Autodesk Inventor part; units mm, degrees
ref_plane "YZ Plane" through (0, 0, 0) normal (1, 0, 0) x (0, 1, 0)
ref_plane "XZ Plane" through (0, 0, 0) normal (0, 1, 0) x (-1, 0, 0)
ref_plane "XY Plane" through (0, 0, 0) normal (0, 0, 1) x (1, 0, 0)
sketch "Sketch1" plane through (0, 0, 0) normal (1, 0, 0) x (0, 1, 0)
  arc A0 (19.1422, -3.9768) -> (18.6646, -2.8408) centre (18.6646, -3.5092) ccw
  line L0 (15.9535, -7.2342) -> (19.1422, -3.9768)
  line L1 (21.0667, -5.7702) -> (17.9387, -8.9655)
  arc A1 (22.2128, -6.2377) -> (21.0667, -5.7702) centre (21.5444, -6.2377) ccw
  line L2 (25.0536, -2.0053) -> (25.0536, -8.7443)
  line L3 (22.2128, -8.7443) -> (22.2128, -6.2377)
  line L4 (-0.0122, -2.0053) -> (-0.0122, -8.7443)
  arc A2 (3.9747, -5.7702) -> (2.8286, -6.2377) centre (3.497, -6.2377) ccw
  arc A3 (1.9931, 0) -> (-0.0122, -2.0053) centre (1.9931, -2.0053) ccw
  line L5 (8.8992, 0) -> (1.9931, 0)
  arc A4 (7.1027, -16.4345) -> (8.0089, -14.2135) centre (4.8339, -14.2135) ccw
  arc A5 (18.6646, -22.5592) -> (19.1422, -21.4232) centre (18.6646, -21.8908) ccw
  line L6 (15.9535, -18.1658) -> (19.1422, -21.4232)
  arc A6 (21.0667, -19.6298) -> (22.2128, -19.1623) centre (21.5444, -19.1623) ccw
  line L7 (21.0667, -19.6298) -> (17.9387, -16.4345)
  line L8 (22.2128, -16.6557) -> (22.2128, -19.1623)
  line L9 (25.0536, -23.3947) -> (25.0536, -16.6557)
  line L10 (16.1422, 0) -> (23.0483, 0)
  line L11 (18.6646, -2.8408) -> (16.0299, -2.8408)
  arc A7 (22.2128, -8.7443) -> (23.3277, -9.8592) centre (23.3277, -8.7443) ccw
  line L12 (23.9387, -9.8592) -> (23.3277, -9.8592)
  arc A8 (23.9387, -9.8592) -> (25.0536, -8.7443) centre (23.9387, -8.7443) ccw
  arc A9 (6.3768, -2.8408) -> (5.8991, -3.9768) centre (6.3768, -3.5092) ccw
  line L13 (3.9747, -5.7702) -> (7.1027, -8.9655)
  line L14 (9.0879, -7.2342) -> (5.8991, -3.9768)
  arc A10 (2.8286, -19.1623) -> (3.9747, -19.6298) centre (3.497, -19.1623) ccw
  line L15 (-0.0122, -23.3947) -> (-0.0122, -16.6557)
  line L16 (3.9747, -19.6298) -> (7.1027, -16.4345)
  arc A11 (5.8991, -21.4232) -> (6.3768, -22.5592) centre (6.3768, -21.8908) ccw
  line L17 (9.0879, -18.1658) -> (5.8991, -21.4232)
  line L18 (2.8286, -16.6557) -> (2.8286, -19.1623)
  arc A12 (23.0483, -25.4) -> (25.0536, -23.3947) centre (23.0483, -23.3947) ccw
  arc A13 (25.0536, -2.0053) -> (23.0483, 0) centre (23.0483, -2.0053) ccw
  arc A14 (13.6846, -8.1882) -> (15.9535, -7.2342) centre (13.6846, -5.0132) ccw
  line L19 (13.6846, -8.1882) -> (11.3567, -8.1882)
  arc A15 (9.0115, -2.8408) -> (10.0141, -1.8382) centre (9.0115, -1.8382) ccw
  arc A16 (9.0879, -7.2342) -> (11.3567, -8.1882) centre (11.3567, -5.0132) ccw
  arc A17 (17.9387, -8.9655) -> (17.0325, -11.1865) centre (20.2075, -11.1865) ccw
  line L20 (17.0325, -14.2135) -> (17.0325, -11.1865)
  line L21 (6.3768, -2.8408) -> (9.0115, -2.8408)
  line L22 (10.0141, -1.8382) -> (10.0141, -1.1149)
  arc A18 (10.0141, -1.1149) -> (8.8992, 0) centre (8.8992, -1.1149) ccw
  line L23 (2.8286, -8.7443) -> (2.8286, -6.2377)
  arc A19 (1.7137, -9.8592) -> (2.8286, -8.7443) centre (1.7137, -8.7443) ccw
  line L24 (1.1027, -9.8592) -> (1.7137, -9.8592)
  arc A20 (-0.0122, -8.7443) -> (1.1027, -9.8592) centre (1.1027, -8.7443) ccw
  line L25 (6.3768, -22.5592) -> (9.0115, -22.5592)
  arc A21 (10.0141, -23.5618) -> (9.0115, -22.5592) centre (9.0115, -23.5618) ccw
  line L26 (10.0141, -23.5618) -> (10.0141, -24.2851)
  arc A22 (8.8992, -25.4) -> (10.0141, -24.2851) centre (8.8992, -24.2851) ccw
  line L27 (8.8992, -25.4) -> (1.9931, -25.4)
  arc A23 (17.0325, -14.2135) -> (17.9387, -16.4345) centre (20.2075, -14.2135) ccw
  line L28 (23.9387, -15.5408) -> (23.3277, -15.5408)
  arc A24 (23.3277, -15.5408) -> (22.2128, -16.6557) centre (23.3277, -16.6557) ccw
  arc A25 (25.0536, -16.6557) -> (23.9387, -15.5408) centre (23.9387, -16.6557) ccw
  line L29 (16.1422, -25.4) -> (23.0483, -25.4)
  line L30 (18.6646, -22.5592) -> (16.0299, -22.5592)
  line L31 (8.0089, -11.1865) -> (8.0089, -14.2135)
  arc A26 (8.0089, -11.1865) -> (7.1027, -8.9655) centre (4.8339, -11.1865) ccw
  arc A27 (15.0273, -1.8382) -> (16.0299, -2.8408) centre (16.0299, -1.8382) ccw
  line L32 (15.0273, -1.8382) -> (15.0273, -1.1149)
  arc A28 (16.1422, 0) -> (15.0273, -1.1149) centre (16.1422, -1.1149) ccw
  arc A29 (-0.0122, -23.3947) -> (1.9931, -25.4) centre (1.9931, -23.3947) ccw
  arc A30 (11.3567, -17.2118) -> (9.0879, -18.1658) centre (11.3567, -20.3868) ccw
  line L33 (11.3567, -17.2118) -> (13.6846, -17.2118)
  arc A31 (15.9535, -18.1658) -> (13.6846, -17.2118) centre (13.6846, -20.3868) ccw
  arc A32 (16.0299, -22.5592) -> (15.0273, -23.5618) centre (16.0299, -23.5618) ccw
  line L34 (15.0273, -23.5618) -> (15.0273, -24.2851)
  arc A33 (15.0273, -24.2851) -> (16.1422, -25.4) centre (16.1422, -24.2851) ccw
  line L35 (1.1027, -15.5408) -> (1.7137, -15.5408)
  arc A34 (1.1027, -15.5408) -> (-0.0122, -16.6557) centre (1.1027, -16.6557) ccw
  arc A35 (2.8286, -16.6557) -> (1.7137, -15.5408) centre (1.7137, -16.6557) ccw
  point P0 (0, 0)
  point P1 (12.5207, -12.7)
  dimension "d0" = 25.4
extrude "Extrusion1" add sketch "Sketch1" along normal blind 101.6
properties part number "extruded aluminum"
Model file for the job. Use its own axes, mm. A direction names the side the tool comes from. Coordinates: 2 decimals unless noted, no trailing zeros. Write each loop counter-clockwise with the first axis right and the second up, starting at its lowest first coordinate (ties: lowest second). Pieces come first, ordered by that corner, then holes. Notation, with made-up numbers: (69, -22.5) - (119, -22.5) arc R10 cw to (119, -10.5) - close; hole circle Ø11 at (-28.75, 16). An arc over 180 degrees is marked (long way). One line per question, with ' | ' between items. Start each with the question number.
Q1. Pull direction Z, two halves, no side cores. Call faces 4 (the face through (50, 20, -25.4)), 5 (the face through (50, -0.012, -20)), 6 (the face through (50.09, 19.52, -7.35)): pulls with the +Z half, pulls with the -Z half, needs draft (parallel to the pull), parting line crosses it, or undercut.
Q2. Cut at A-A, the plane z = -12.25. List the corners of the cut face in (x, y), then the cut area to 3 significant figures.
Q3. Drill centre lines: line 1 (Z direction, x = 5.5, y = 3.5); line 2 (Z direction, x = 43, y = 7.5); line 3 (Z direction, x = 73.5, y = 16.25). Where is each one in solid material? Low to high. Write a range as [from, to].
Q4. 3-axis set-ups, long thin cutter, end or side, ignore diameter. For faces 1 (the face through (50, 17.032, -13)), 2 (the face through (50, 13, -17.212)), 3 (the face through (50.089, 17.274, -15.429)): which of +Z, -Z, +X, -X, +Y, -Y reach the whole face in a straight line?
Q5. Pin check, flat tips, straight feed: pin 1 (0.6 mm diameter, centred on x = 58.5, z = -1.5, fed in from -Y); pin 2 (2.5 mm diameter, centred on x = 69, z = -13, fed in from -Y); pin 3 (0.5 mm diameter, centred on x = 59, y = 23.5, fed in from -Z). Stop position of each tip, or through.
Answer below:
1) face 4: pulls with the -Z half | face 5: needs draft | face 6: undercut
2) outline: (0, 8.01) - (101.6, 8.01) - (101.6, 17.03) - (0, 17.03) - close | area: 917 mm^2
3) line 1: [-25.4, -19.83], [-5.57, 0] | line 2: [-25.4, -22.56], [-19.79, -15.94], [-9.46, -5.61], [-2.84, 0] | line 3: [-25.4, -22.56], [-18.47, -6.93], [-2.84, 0]
4) face 1: +X, -X, +Y | face 2: -Z, +X, -X | face 3: +X, -X
5) pin 1: y = 0 | pin 2: y = 8.01 | pin 3: z = -25.39
